Input: part model. Units: mm. Frame: model coordinates. Round coordinates to 2 decimals unless told otherwise and drop trailing zeros. Loops run counter-clockwise (first coordinate to the right, second up) from the corner with the lowest first, then second, coordinate; pieces in that order, holes last.
(1) Line query: line 1 (Y direction, x = -12.7, z = -1.7) (3 decimals); line 2 (X direction, y = 209.5, z = -1.5); line 3 (Y direction, x = 48.5, z = -2.1). Output: solid intervals per line, ascending.
(2) Cut plane B-B, the plane z = -1.3. Give the number of separate pieces and of enclosed holes in the cut face, and give its area (3 significant figures).
(3) First-contact query: pin 1 Ø6 at (x, y) = (165.89, 230.17) entering from +Z; pin 2 Ø1 at (x, z) = (48.5, -2) entering from -Y. Flat tips, straight axial feed; report the tip coordinate or a pass-through.
(4) Cut plane C-C, the plane x = 23. Output: boundary loops of the cut face in (y, z) (3 decimals), and give its area (3 significant figures).
(5) Cut plane D-D, the plane y = 175.5. Output: boundary loops of the cut face in (x, z) (3 decimals).
(6) Draft query along Y for faces 1 (the face through (193.65, 235.21, -1.57)), 2 (the face through (-8, 112, -3.175)), 3 (the face through (175.94, 223.716, -1.565)). Return one class per face: released by +Y, released by -Y, zero draft, split by the parting line, or undercut.
(7) Cut plane A-A, the plane x = 177.8. Output: boundary loops of the cut face in (y, z) (1 decimal), and give its area (3 significant figures).
from build123d import *

# Parameters (mm, degrees)
SKETCH1_R          = 3.175
SKETCH1_R_2        = 14.2875
SKETCH1_R_3        = 2.54
BASE_FLANGE1_DEPTH = 3.175


# Sheet-metal steps are written as plain solids
with BuildPart() as part:
    # Sketch1 → Base-Flange1 (new body)
    with BuildSketch(Plane.XY):
        with BuildLine():
            Line((0, 0), (-127, 0))
            Line((-127, 0), (-127, 25.4))
            ThreePointArc((-127, 25.4), (-52.707547813, 97.203546852), (-25.4, 196.85))
            Line((-25.4, 196.85), (0, 196.85))
            Line((0, 196.85), (106.3625, 196.85))
            ThreePointArc((106.3625, 196.85), (132.498884376, 204.089359374), (151.186029412, 223.744117647))
            ThreePointArc((151.186029412, 223.744117647), (194.239231655, 234.838892203), (201.574896344, 190.988461538))
            ThreePointArc((201.574896344, 190.988461538), (183.810239349, 176.595174659), (161.532965659, 171.45))
            Line((161.532965659, 171.45), (0, 171.45))
            Line((0, 171.45), (0, 0))
        make_face()
        with Locations((-12.7, 12.7)):
            Circle(SKETCH1_R, mode=Mode.SUBTRACT)
        with Locations((-12.7, 184.15)):
            Circle(SKETCH1_R, mode=Mode.SUBTRACT)
        with Locations((-114.3, 12.7)):
            Circle(SKETCH1_R, mode=Mode.SUBTRACT)
        with Locations((-63.5, 12.7)):
            Circle(SKETCH1_R, mode=Mode.SUBTRACT)
        with Locations((-12.7, 98.425)):
            Circle(SKETCH1_R, mode=Mode.SUBTRACT)
        with Locations((177.8, 209.55)):
            Circle(SKETCH1_R_2, mode=Mode.SUBTRACT)
        with Locations((201.6125, 209.55)):
            Circle(SKETCH1_R_3, mode=Mode.SUBTRACT)
        with Locations((189.70625, 188.927770072)):
            Circle(SKETCH1_R_3, mode=Mode.SUBTRACT)
        with Locations((165.89375, 188.927770072)):
            Circle(SKETCH1_R_3, mode=Mode.SUBTRACT)
        with Locations((153.9875, 209.55)):
            Circle(SKETCH1_R_3, mode=Mode.SUBTRACT)
        with Locations((165.89375, 230.172229928)):
            Circle(SKETCH1_R_3, mode=Mode.SUBTRACT)
        with Locations((189.70625, 230.172229928)):
            Circle(SKETCH1_R_3, mode=Mode.SUBTRACT)
        with Locations((66.675, 184.15)):
            Circle(SKETCH1_R, mode=Mode.SUBTRACT)
        with Locations((-12.7, 158.75)):
            Circle(SKETCH1_R, mode=Mode.SUBTRACT)
        with Locations((146.05, 184.15)):
            Circle(SKETCH1_R, mode=Mode.SUBTRACT)
    extrude(amount=-BASE_FLANGE1_DEPTH)


solid = part.part
Reported:
1. line 1: y = 0 to 9.525, 15.875 to 95.25, 101.6 to 155.575, 161.925 to 180.975, 187.325 to 196.85
1. line 2: x = 139.91 to 151.45, 156.53 to 163.51, 192.09 to 199.07, 204.15 to 207.96
1. line 3: y = 171.45 to 196.85
2. separate pieces: 1
2. enclosed holes: 15
2. area: 18,900 mm2
3. pin 1: stops at z = 0
3. pin 2: stops at y = 171.45
4. outline: (171.45, -3.175) - (196.85, -3.175) - (196.85, 0) - (171.45, 0) - close
4. area: 80.6 mm2
5. outline: (-26.57, -3.175) - (181.41, -3.175) - (181.41, 0) - (-26.57, 0) - close
6. face 1: split by the parting line
6. face 2: zero draft
6. face 3: undercut
7. outline: (174.1, -3.2) - (195.3, -3.2) - (195.3, 0) - (174.1, 0) - close; (223.8, -3.2) - (239.7, -3.2) - (239.7, 0) - (223.8, 0) - close
7. area: 118 mm2
